from build123d import *

# Parameters (mm, degrees)
SKETCH1_R           = 12.5
BOSS_EXTRUDE2_DEPTH = 15
CUT_EXTRUDE1_REACH  = 36.821
CHAMFER1_SIZE       = 2
FILLET1_R           = 1


with BuildPart() as part:
    # Sketch1 → Boss-Extrude2 (new body)
    with BuildSketch(Plane(origin=(0, 0, 0), x_dir=(1, 0, 0), z_dir=(0, 1, 0))):
        with Locations(Location((0, 0, 0), (0, 0, 270))):
            Circle(SKETCH1_R)
    extrude(amount=BOSS_EXTRUDE2_DEPTH)

    # Sketch2 → Revolve1 (revolve)
    with BuildSketch(Plane.XY):
        Polygon((12.5, 15), (0, 30), (0, 15), align=None)
    revolve(axis=Axis((0, -1000, 0), (0, 1, 0)))

    # Cut-Extrude1: up to this cone (the profile starts inside it)
    cut_extrude1_end = Plane(origin=(0, 0, 0), z_dir=(0, -1, 0)).offset(-29.999999) * Cone(1e-06, 76.934166667, 92.320999, align=(Align.CENTER, Align.CENTER, Align.MIN), mode=Mode.PRIVATE)
    # Sketch3 → Cut-Extrude1 (cut, up to the surface)
    with BuildSketch(Plane(origin=(0, 0, 0), x_dir=(1, 0, 0), z_dir=(0, 1, 0)), mode=Mode.PRIVATE) as cut_extrude1_sk1:
        with BuildLine():
            Line((-10, 7.5), (-10, -7.5))
            ThreePointArc((-10, -7.5), (-12.5, 0), (-10, 7.5))
        make_face()
    cut_extrude1_tool1 = extrude(cut_extrude1_sk1.sketch, amount=CUT_EXTRUDE1_REACH, mode=Mode.PRIVATE) & cut_extrude1_end
    add(cut_extrude1_tool1.solids().sort_by_distance((-11.0091, 0, 0))[0], mode=Mode.SUBTRACT)
    # Sketch3 → Cut-Extrude1 (cut, up to the surface)
    with BuildSketch(Plane(origin=(0, 0, 0), x_dir=(1, 0, 0), z_dir=(0, 1, 0)), mode=Mode.PRIVATE) as cut_extrude1_sk2:
        with BuildLine():
            Line((10, 7.5), (10, -7.5))
            ThreePointArc((10, -7.5), (12.5, 0), (10, 7.5))
        make_face()
    cut_extrude1_tool2 = extrude(cut_extrude1_sk2.sketch, amount=CUT_EXTRUDE1_REACH, mode=Mode.PRIVATE) & cut_extrude1_end
    add(cut_extrude1_tool2.solids().sort_by_distance((11.0091, 0, 0))[0], mode=Mode.SUBTRACT)

    # Chamfer1
    chamfer1_edges = [part.edges().sort_by_distance(p)[0] for p in [
        (0, 0, -12.5),
        (0, 0, 12.5),
        (-10, 0, 0),
        (10, 0, 0),
    ]]
    chamfer(chamfer1_edges, length=CHAMFER1_SIZE)

    # Fillet1
    fillet1_edges = [part.edges().sort_by_distance(p)[0] for p in [
        (-10, 17.087815774, 3.972518962),
        (10, 17.087815774, -3.972518962),
        (0, 15, -12.5),
        (0, 15, 12.5),
    ]]
    fillet(fillet1_edges, radius=FILLET1_R)


solid = part.part
Build history of the part. All positions in model axes, mm. Round coordinates to 2 decimals unless told otherwise and drop trailing zeros. Write each loop counter-clockwise with the first axis right and the second up, starting at its lowest first coordinate (ties: lowest second). Pieces come first, ordered by that corner, then holes. Notation, with made-up numbers: (81.25, 55) - (136.25, 55) arc R29 cw to (136.25, 76) - close; hole circle Ø10 at (79.25, 59.5). An arc over 180 degrees is marked (long way). One line per question, with ' | ' between items.
1. Drop a flat-ended pin along its axis: pin 1 Ø5 at (x, z) = (-1.5, 9) entering from +Y. Give the stop position or say it passes through.
Results are:
pin 1: y = 22.05
2. Band-saw the part on B-B, the plane y = 20.5. Write the cut outline in (x, z).
Results are:
outline: circle Ø15.83 at (0, 0)
3. Drill centre lines: line 1 along X through (y, z) = (11, 10); line 2 along Z through (x, y) = (0.25, 27); line 3 along Y through (x, z) = (7.75, -7.25) (1 decimal). Where is each one in solid material? Low to high. Write a range as from..to.
Results are:
line 1: -7.5..7.5 | line 2: -2.49..2.49 | line 3: 0.1..17.3
4. Band-saw the part on A-A, the plane y = 3.5. Write the cut outline in (x, z), and give its area (3 significant figures).
Results are:
outline: (-10, -7.5) arc R12.5 ccw to (10, -7.5) - (10, 7.5) arc R12.5 ccw to (-10, 7.5) - close | area: 440 mm^2
